Part model, mm, in its own coordinate system. A direction names the side the tool comes from. Give positions to 0.01 mm unless a question says otherwise; leave off trailing zeros. Loops run counter-clockwise (first coordinate to the right, second up) from the corner with the lowest first, then second, coordinate; pieces in that order, holes last. Notation, with made-up numbers: (-8, 38.5) -> (3, 38.5) arc R20 cw to (3, 42.5) -> close; hole circle Ø4 at (12, 16). An arc over 180 degrees is marked (long way). Write item = value, one per line.
from build123d import *

# Parameters (mm, degrees)
SKETCH1_R                = 17
BOSS_EXTRUDE1_DEPTH      = 6
SKETCH2_R                = 33
SKETCH2_R_2              = 21
CUT_EXTRUDE1_DEPTH       = 2
SKETCH3_R                = 5.5
CUT_EXTRUDE2_DEPTH       = 1
CUT_EXTRUDE2_DEPTH_BACK  = 7
M6_CLEARANCE_HOLE1_D     = 6.6
M6_CLEARANCE_HOLE1_DEPTH = 4
CIRPATTERN1_COUNT        = 6


with BuildPart() as part:
    # Sketch1 → Boss-Extrude1 (new body)
    with BuildSketch(Plane(origin=(0, 0, 0), x_dir=(1, 0, 0), z_dir=(0, 1, 0))):
        with BuildLine():
            Line((-50, -65), (50, -65))
            ThreePointArc((50, -65), (60.606601718, -60.606601718), (65, -50))
            Line((65, -50), (65, 50))
            ThreePointArc((65, 50), (60.606601718, 60.606601718), (50, 65))
            Line((50, 65), (-50, 65))
            ThreePointArc((-50, 65), (-60.606601718, 60.606601718), (-65, 50))
            Line((-65, 50), (-65, -50))
            ThreePointArc((-65, -50), (-60.606601718, -60.606601718), (-50, -65))
        make_face()
        Circle(SKETCH1_R, mode=Mode.SUBTRACT)
    extrude(amount=BOSS_EXTRUDE1_DEPTH)

    # Sketch2 → Cut-Extrude1 (cut)
    with BuildSketch(Plane(origin=(0, 6, 0), x_dir=(1, 0, 0), z_dir=(0, 1, 0))):
        Circle(SKETCH2_R)
        Circle(SKETCH2_R_2, mode=Mode.SUBTRACT)
    extrude(amount=-CUT_EXTRUDE1_DEPTH, mode=Mode.SUBTRACT)

    # Sketch3 → Cut-Extrude2 (cut, two sides)
    with BuildSketch(Plane(origin=(0, 6, 0), x_dir=(1, 0, 0), z_dir=(0, 1, 0))) as cut_extrude2_sk:
        with Locations((-50, 50)):
            Circle(SKETCH3_R)
        with Locations((50, 50)):
            Circle(SKETCH3_R)
        with Locations((50, -50)):
            Circle(SKETCH3_R)
        with Locations((-50, -50)):
            Circle(SKETCH3_R)
    extrude(amount=CUT_EXTRUDE2_DEPTH, mode=Mode.SUBTRACT)
    extrude(cut_extrude2_sk.sketch, amount=-CUT_EXTRUDE2_DEPTH_BACK, mode=Mode.SUBTRACT)

    # M6 Clearance Hole1
    with Locations(Plane(origin=(-27, 4, 0), x_dir=(0, 0, 1), z_dir=(0, 1, 0))):
        with Locations((0, 0)):
            m6_clearance_hole1 = Hole(M6_CLEARANCE_HOLE1_D / 2, depth=M6_CLEARANCE_HOLE1_DEPTH)

    # CirPattern1: M6 Clearance Hole1 ×6 about axis
    cirpattern1_axis = Axis((0, 0, 0), (0, 1, 0))
    for i in range(1, CIRPATTERN1_COUNT):
        add(m6_clearance_hole1.rotate(cirpattern1_axis, i * 360 / CIRPATTERN1_COUNT), mode=Mode.SUBTRACT)


solid = part.part
1) Slice it at D-D, the plane y = 0.95. Count the separate pieces of the cut face and the enclosed holes in it, and give its area (3 significant figures).
Resolved:
separate_pieces = 1
enclosed_holes = 11
area = 15,200 mm²
2) Slice it at A-A, the plane x = -27. List the corners of the cut face in (y, z).
Resolved:
outline = (0, -65) -> (6, -65) -> (6, -18.97) -> (4, -18.97) -> (4, -3.3) -> (0, -3.3) -> close; (0, 3.3) -> (4, 3.3) -> (4, 18.97) -> (6, 18.97) -> (6, 65) -> (0, 65) -> close
3) Drill centre lines: line 1 along X through (y, z) = (2.05, -50); line 2 along X through (y, z) = (2.25, 0). Where is each one in solid material? Low to high. Write a range as [from, to].
Resolved:
line_1 = [-65, -55.5], [-44.5, 44.5], [55.5, 65]
line_2 = [-65, -30.3], [-23.7, -17], [17, 23.7], [30.3, 65]
4) Slice it at B-B, the plane x = -48. List the corners of the cut face in (y, z), and give its area (3 significant figures).
Resolved:
outline = (0, -65) -> (6, -65) -> (6, -55.12) -> (0, -55.12) -> close; (0, -44.88) -> (6, -44.88) -> (6, 44.88) -> (0, 44.88) -> close; (0, 55.12) -> (6, 55.12) -> (6, 65) -> (0, 65) -> close
area = 657 mm²
5) Drop a flat-ended pin along its axis: P1, Ø6, axis at x = -13.5, z = 23.38, coming from the +Y side. Give the stop position or say it passes through.
Resolved:
P1 = through
6) Which spindle directions (+Z, -Z, +X, -X, +Y, -Y) get a long thin tool onto all of the face, cutting with end or side? Do faces 5 (the face through (9.139, 2.958, -14.334)), 6 (the face through (30.5, 5, 12.6)). Say none if no direction does.
Resolved:
face_5 = +Y, -Y
face_6 = +Y
7) Slice it at C-C, the plane z = -13. List the corners of the cut face in (x, y), and give its area (3 significant figures).
Resolved:
outline = (-65, 0) -> (-10.95, 0) -> (-10.95, 6) -> (-16.49, 6) -> (-16.49, 4) -> (-30.33, 4) -> (-30.33, 6) -> (-65, 6) -> close; (10.95, 0) -> (65, 0) -> (65, 6) -> (30.33, 6) -> (30.33, 4) -> (16.49, 4) -> (16.49, 6) -> (10.95, 6) -> close
area = 593 mm²
8) Pull direction X, two halves, no side cores. Call faces 1 (the face through (-12.236, 1.972, 26.431)), 2 (the face through (22, 4, 0)), 3 (the face through (-15, 0, -15)), 4 (the face through (60.49, 2.96, 60.72)): pulls with the +X half, pulls with the -X half, needs draft (parallel to the pull), parting line crosses it, or undercut.
Resolved:
face_1 = undercut
face_2 = undercut
face_3 = needs draft
face_4 = pulls with the +X half
